Geometry check sheet. Reference: drawing and pictorial views, mm from the part's lowest x, y, z. Round coordinates to 2 decimals unless told otherwise and drop trailing zeros. Write each loop counter-clockwise with the first axis right and the second up, starting at its lowest first coordinate (ties: lowest second). Pieces come first, ordered by that corner, then holes. Notation, with made-up numbers: (79.25, 81.25) -> (97.25, 81.25) arc R21 cw to (97.25, 100.25) -> close; hole circle Ø8 at (44.5, -2.75). An arc over 180 degrees is marked (long way). Answer as a JSON object with one key per item and string values. Group by question number.
(1) Scan lines: L1, parallel to Z at x = 14.4, y = 0.95; L2, parallel to Z at x = 14.4, y = 2.5; L3, parallel to X at y = 2.7, z = 4.2. Record each from-to range of solid material in increasing order. Write a range as from..to.
(2) Gauge pin test, flat ends, axial feed: pin 1 Ø2 at (x, z) = (3.5, 12) entering from -Y; pin 2 Ø1.8 at (x, z) = (13.5, 3.5) entering from -Y. Record the tip position at first contact, or that the pin passes through.
(3) Sectioned sample at A-A on x = 13.5. Record the cut outline in (y, z), and give its area (3 significant figures).
(4) Sectioned sample at C-C on z = 24.2. Record the cut outline in (x, y).
(5) Sectioned sample at B-B on y = 1.7. Record the cut outline in (x, z), and give its area (3 significant figures).
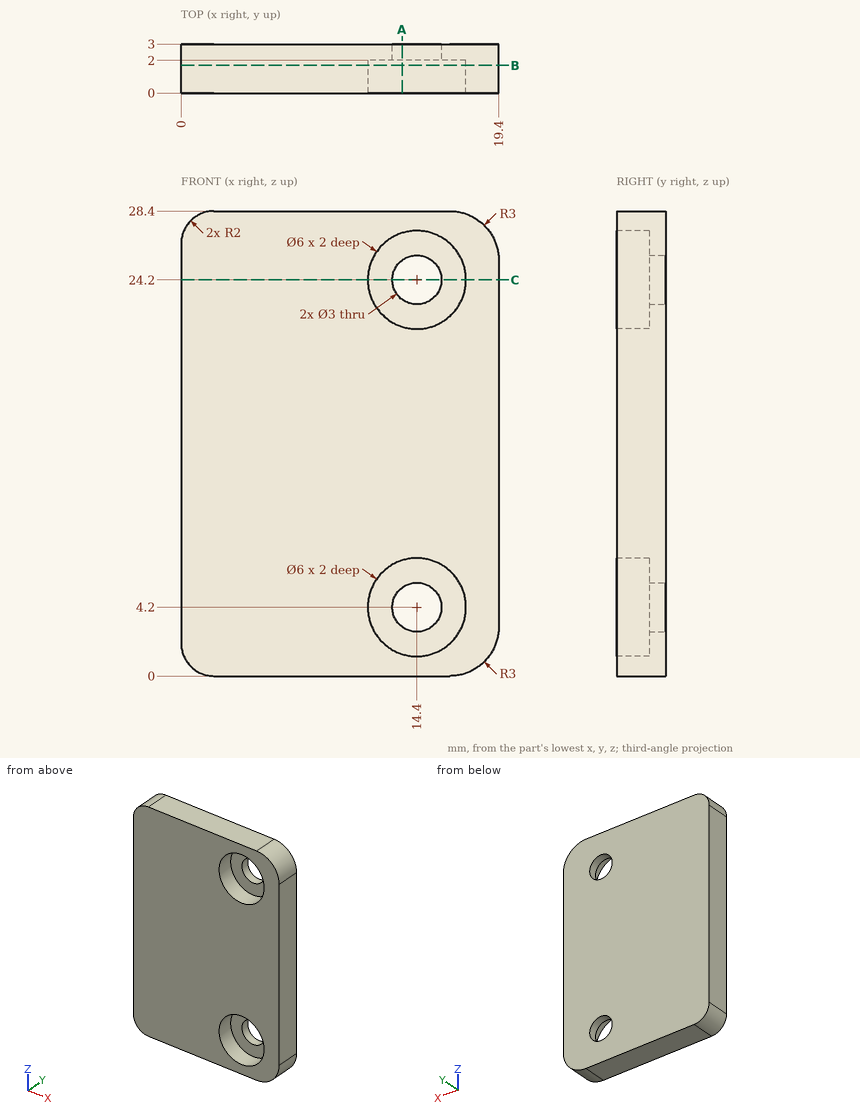
Computed values:
{
 "1": {"L1": "0..1.2, 7.2..21.2, 27.2..28.4", "L2": "0..2.7, 5.7..22.7, 25.7..28.4", "L3": "0..12.9, 15.9..19.4"},
 "2": {"pin 1": "y = 0", "pin 2": "y = 2"},
 "3": {"outline": "(0, 0) -> (3, 0) -> (3, 3) -> (2, 3) -> (2, 1.34) -> (0, 1.34) -> close; (0, 7.06) -> (2, 7.06) -> (2, 5.4) -> (3, 5.4) -> (3, 23) -> (2, 23) -> (2, 21.34) -> (0, 21.34) -> close; (0, 27.06) -> (2, 27.06) -> (2, 25.4) -> (3, 25.4) -> (3, 28.4) -> (0, 28.4) -> close", "area": "57.5 mm2"},
 "4": {"outline": "(0, 0) -> (11.4, 0) -> (11.4, 2) -> (12.9, 2) -> (12.9, 3) -> (0, 3) -> close; (15.9, 2) -> (17.4, 2) -> (17.4, 0) -> (19.4, 0) -> (19.4, 3) -> (15.9, 3) -> close"},
 "5": {"outline": "(0, 2) arc R2 ccw to (2, 0) -> (16.4, 0) arc R3 ccw to (19.4, 3) -> (19.4, 25.4) arc R3 ccw to (16.4, 28.4) -> (2, 28.4) arc R2 ccw to (0, 26.4) -> close; hole circle Ø6 at (14.4, 4.2); hole circle Ø6 at (14.4, 24.2)", "area": "489 mm2"}
}
